Study the drawing (mm; zero at the part's minimum x, y, z) and answer. Coordinates: 2 decimals unless noted, no trailing zeros. Loops run counter-clockwise (first coordinate to the right, second up) from the corner with the lowest first, then second, coordinate; pieces in that order, holes last. Notation, with made-up numbers: (26.5, -37) -> (84.5, -37) arc R25 cw to (84.5, 0) -> close; hole circle Ø8 at (72, 57). An arc over 180 degrees is marked (long way). Answer in a Markdown table with one row per item.
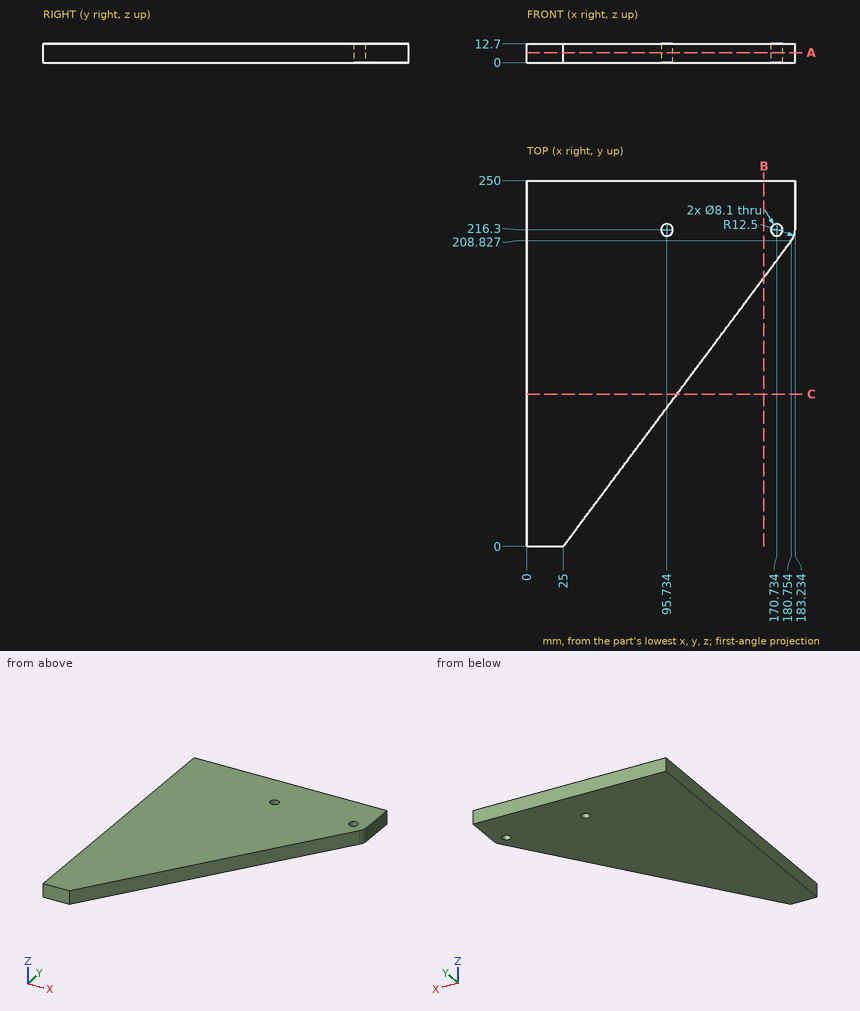
1. A cutting plane is placed at B-B on x = 162. Give the vertices of the cut face in (y, z).
A:
| item | result |
|---|---|
| outline | (183.68, 0) -> (250, 0) -> (250, 12.7) -> (183.68, 12.7) -> close |
2. A cutting plane is placed at A-A on z = 6.75. Give the vertices of the cut face in (x, y), and give its area (3 significant figures).
A:
| item | result |
|---|---|
| outline | (0, 0) -> (25, 0) -> (180.75, 208.83) arc R12.5 ccw to (183.23, 216.3) -> (183.23, 250) -> (0, 250) -> close; hole circle Ø8.1 at (95.73, 216.3); hole circle Ø8.1 at (170.73, 216.3) |
| area | 28,900 mm2 |
3. A cutting plane is placed at C-C on y = 104. Give the vertices of the cut face in (x, z).
A:
| item | result |
|---|---|
| outline | (0, 0) -> (102.57, 0) -> (102.57, 12.7) -> (0, 12.7) -> close |
4. Given pin 1 Ø6 at (y, z) = (208.5, 10.5) entering from +X (1 decimal); pin 2 Ø2 at (y, z) = (111.5, 9.5) entering from +X, each flat-ended and moving along its own axis, determine where each tip first touches the part or whether it passes through.
A:
| item | result |
|---|---|
| pin 1 | stops at x = 182.3 |
| pin 2 | stops at x = 108.91 |
5. Find the intervals of material crossed by probe 1 along X at (y, z) = (28.5, 5.25) (1 decimal); probe 2 along Y at (x, z) = (33, 6.5) (1 decimal); probe 3 along X at (y, z) = (32, 2), in increasing order.
A:
| item | result |
|---|---|
| probe 1 | x = 0 to 46.3 |
| probe 2 | y = 10.7 to 250 |
| probe 3 | x = 0 to 48.87 |
